Work out the finished part from the listing and answer in its coordinate system (mm). Face numbers are marked on the shaded views. Give positions to 0.01 mm unless a question says otherwise; leave off trailing zeros. Loops run counter-clockwise (first coordinate to the right, second up) from the corner with the lowest first, then second, coordinate; pieces in that order, holes last.
```python
from build123d import *

# Parameters (mm, degrees)
BOX028_W          = 10
BOX028_H          = 10
BOX028_DEPTH      = 3.5
FILLET018_R       = 1.7
BOX029_W          = 20
BOX029_H          = 10
BOX029_DEPTH      = 3.5
FILLET019_R       = 1.7
CYLINDER029_R     = 5
CYLINDER029_DEPTH = 10
CYLINDER027_R     = 0.25
CYLINDER027_DEPTH = 10
CYLINDER026_R     = 1.75
CYLINDER026_DEPTH = 10
BOX023_W          = 6.65
BOX023_H          = 8.3
BOX023_DEPTH      = 2.45
FILLET014_R       = 1
CYLINDER022_R     = 0.5
CYLINDER022_DEPTH = 10
CYLINDER023_R     = 0.5
CYLINDER023_DEPTH = 10
CYLINDER024_R     = 0.5
CYLINDER024_DEPTH = 10
CYLINDER021_R     = 0.5
CYLINDER021_DEPTH = 10
CYLINDER020_R     = 0.5
CYLINDER020_DEPTH = 10
CYLINDER019_R     = 0.5
CYLINDER019_DEPTH = 10
CYLINDER018_R     = 0.5
CYLINDER018_DEPTH = 10
CYLINDER017_R     = 0.5
CYLINDER017_DEPTH = 10
CYLINDER016_R     = 0.5
CYLINDER016_DEPTH = 10
CYLINDER015_R     = 0.5
CYLINDER015_DEPTH = 10
CYLINDER014_R     = 0.5
CYLINDER014_DEPTH = 10
CYLINDER013_R     = 0.5
CYLINDER013_DEPTH = 10
BOX021_W          = 8
BOX021_H          = 4
BOX021_DEPTH      = 10
FILLET012_R       = 1.5
BOX019_W          = 8
BOX019_H          = 8
BOX019_DEPTH      = 10
FILLET010_R       = 3
BOX001_W          = 133
BOX001_H          = 63
BOX001_DEPTH      = 10
FILLET002_R       = 1
BOX_W             = 137
BOX_H             = 67
BOX_DEPTH         = 7.5
FILLET_R          = 3
FILLET001_R       = 2


with BuildPart() as fillet018:
    # Box028 → Box028 (new body)
    with BuildSketch(Plane(origin=(57, 60, 2.5), x_dir=(1, 0, 0), z_dir=(0, 0, 1))):
        with Locations((5, 5)):
            Rectangle(BOX028_W, BOX028_H)
    extrude(amount=BOX028_DEPTH)

    # Fillet018
    fillet018_edges = [fillet018.edges().sort_by_distance(p)[0] for p in [
        (57, 65, 6),
        (57, 65, 2.5),
        (67, 65, 6),
        (67, 65, 2.5),
    ]]
    fillet(fillet018_edges, radius=FILLET018_R)


with BuildPart() as fillet018_1:
    # Fillet018 placement: moved
    add(fillet018.part.moved(Location((0, 0, -0.6))))


with BuildPart() as fillet019:
    # Box029 → Box029 (new body)
    with BuildSketch(Plane(origin=(57, 60, 2.5), x_dir=(1, 0, 0), z_dir=(0, 0, 1))):
        with Locations((10, 5)):
            Rectangle(BOX029_W, BOX029_H)
    extrude(amount=BOX029_DEPTH)

    # Fillet019
    fillet019_edges = [fillet019.edges().sort_by_distance(p)[0] for p in [
        (57, 65, 6),
        (57, 65, 2.5),
        (77, 65, 6),
        (77, 65, 2.5),
    ]]
    fillet(fillet019_edges, radius=FILLET019_R)


with BuildPart() as fillet019_1:
    # Fillet019 placement: moved
    add(fillet019.part.moved(Location((-25, 0, -0.6))))


with BuildPart() as cilindro027:
    # Cylinder029 → Cylinder029 (new body)
    with BuildSketch(Plane(origin=(37, 33.5, -1), x_dir=(1, 0, 0), z_dir=(0, 0, 1))):
        Circle(CYLINDER029_R)
    extrude(amount=CYLINDER029_DEPTH)


with BuildPart() as cilindro025:
    # Cylinder027 → Cylinder027 (new body)
    with BuildSketch(Plane(origin=(0, 16, 3), x_dir=(0, 1, 0), z_dir=(1, 0, 0))):
        Circle(CYLINDER027_R)
    extrude(amount=CYLINDER027_DEPTH)


with BuildPart() as phones:
    # Cylinder026 → Cylinder026 (new body)
    with BuildSketch(Plane(origin=(-2, 11.75, 3), x_dir=(0, 1, 0), z_dir=(1, 0, 0))):
        Circle(CYLINDER026_R)
    extrude(amount=CYLINDER026_DEPTH)


with BuildPart() as usb_c:
    # Box023 → Box023 (new body)
    with BuildSketch(Plane.XY):
        with Locations((3.325, 4.15)):
            Rectangle(BOX023_W, BOX023_H)
    extrude(amount=BOX023_DEPTH)

    # Fillet014
    fillet014_edges = [usb_c.edges().sort_by_distance(p)[0] for p in [
        (3.325, 0, 0),
        (3.325, 0, 2.45),
        (3.325, 8.3, 0),
        (3.325, 8.3, 2.45),
    ]]
    fillet(fillet014_edges, radius=FILLET014_R)


with BuildPart() as usb_c_1:
    # Fillet014 placement: moved
    add(usb_c.part.moved(Location((132, 29.35, 2.4))))


with BuildPart() as cilindro022:
    # Cylinder022 → Cylinder022 (new body)
    with BuildSketch(Plane(origin=(130, 52.5, 4.25), x_dir=(0, 1, 0), z_dir=(1, 0, 0))):
        Circle(CYLINDER022_R)
    extrude(amount=CYLINDER022_DEPTH)


with BuildPart() as cilindro023:
    # Cylinder023 → Cylinder023 (new body)
    with BuildSketch(Plane(origin=(130, 51, 4.25), x_dir=(0, 1, 0), z_dir=(1, 0, 0))):
        Circle(CYLINDER023_R)
    extrude(amount=CYLINDER023_DEPTH)


with BuildPart() as fusion008:
    # Cylinder024 → Cylinder024 (new body)
    with BuildSketch(Plane(origin=(130, 54, 4.25), x_dir=(0, 1, 0), z_dir=(1, 0, 0))):
        Circle(CYLINDER024_R)
    extrude(amount=CYLINDER024_DEPTH)

    # Fusion009: union Cilindro022, Cilindro023
    add(cilindro022.part)
    add(cilindro023.part)


with BuildPart() as fusion008_1:
    # Fusion009 placement: moved
    add(fusion008.part.moved(Location((0, -33.5, 0))))


with BuildPart() as cilindro021:
    # Cylinder021 → Cylinder021 (new body)
    with BuildSketch(Plane(origin=(130, 52.5, 4.25), x_dir=(0, 1, 0), z_dir=(1, 0, 0))):
        Circle(CYLINDER021_R)
    extrude(amount=CYLINDER021_DEPTH)


with BuildPart() as cilindro020:
    # Cylinder020 → Cylinder020 (new body)
    with BuildSketch(Plane(origin=(130, 51, 4.25), x_dir=(0, 1, 0), z_dir=(1, 0, 0))):
        Circle(CYLINDER020_R)
    extrude(amount=CYLINDER020_DEPTH)


with BuildPart() as agujero_micro:
    # Cylinder019 → Cylinder019 (new body)
    with BuildSketch(Plane(origin=(130, 54, 4.25), x_dir=(0, 1, 0), z_dir=(1, 0, 0))):
        Circle(CYLINDER019_R)
    extrude(amount=CYLINDER019_DEPTH)

    # Fusion008: union Cilindro021, Cilindro020
    add(cilindro021.part)
    add(cilindro020.part)


with BuildPart() as agujero_micro_1:
    # Fusion008 placement: moved
    add(agujero_micro.part.moved(Location((0, -38, 0))))

    # Fusion010: union Fusion008
    add(fusion008_1.part)


with BuildPart() as cilindro018:
    # Cylinder018 → Cylinder018 (new body)
    with BuildSketch(Plane(origin=(130, 52.5, 4.25), x_dir=(0, 1, 0), z_dir=(1, 0, 0))):
        Circle(CYLINDER018_R)
    extrude(amount=CYLINDER018_DEPTH)


with BuildPart() as cilindro017:
    # Cylinder017 → Cylinder017 (new body)
    with BuildSketch(Plane(origin=(130, 51, 4.25), x_dir=(0, 1, 0), z_dir=(1, 0, 0))):
        Circle(CYLINDER017_R)
    extrude(amount=CYLINDER017_DEPTH)


with BuildPart() as fusion006:
    # Cylinder016 → Cylinder016 (new body)
    with BuildSketch(Plane(origin=(130, 54, 4.25), x_dir=(0, 1, 0), z_dir=(1, 0, 0))):
        Circle(CYLINDER016_R)
    extrude(amount=CYLINDER016_DEPTH)

    # Fusion006: union Cilindro018, Cilindro017
    add(cilindro018.part)
    add(cilindro017.part)


with BuildPart() as fusion006_1:
    # Fusion006 placement: moved
    add(fusion006.part.moved(Location((0, -4.5, 0))))


with BuildPart() as cilindro015:
    # Cylinder015 → Cylinder015 (new body)
    with BuildSketch(Plane(origin=(130, 52.5, 4.25), x_dir=(0, 1, 0), z_dir=(1, 0, 0))):
        Circle(CYLINDER015_R)
    extrude(amount=CYLINDER015_DEPTH)


with BuildPart() as cilindro014:
    # Cylinder014 → Cylinder014 (new body)
    with BuildSketch(Plane(origin=(130, 51, 4.25), x_dir=(0, 1, 0), z_dir=(1, 0, 0))):
        Circle(CYLINDER014_R)
    extrude(amount=CYLINDER014_DEPTH)


with BuildPart() as obj1:
    # Cylinder013 → Cylinder013 (new body)
    with BuildSketch(Plane(origin=(130, 54, 4.25), x_dir=(0, 1, 0), z_dir=(1, 0, 0))):
        Circle(CYLINDER013_R)
    extrude(amount=CYLINDER013_DEPTH)

    # Fusion005: union Cilindro015, Cilindro014
    add(cilindro015.part)
    add(cilindro014.part)

    # Fusion007: union Fusion006
    add(fusion006_1.part)


with BuildPart() as fillet012:
    # Box021 → Box021 (new body)
    with BuildSketch(Plane(origin=(4, 55, -1), x_dir=(1, 0, 0), z_dir=(0, 0, 1))):
        with Locations((4, 2)):
            Rectangle(BOX021_W, BOX021_H)
    extrude(amount=BOX021_DEPTH)

    # Fillet012
    fillet012_edges = [fillet012.edges().sort_by_distance(p)[0] for p in [
        (4, 55, 4),
        (4, 59, 4),
        (12, 55, 4),
        (12, 59, 4),
    ]]
    fillet(fillet012_edges, radius=FILLET012_R)


with BuildPart() as fillet012_1:
    # Fillet012 placement: moved
    add(fillet012.part.moved(Location((0, -6, 0))))


with BuildPart() as fillet010:
    # Box019 → Box019 (new body)
    with BuildSketch(Plane(origin=(4, 55, -1), x_dir=(1, 0, 0), z_dir=(0, 0, 1))):
        with Locations((4, 4)):
            Rectangle(BOX019_W, BOX019_H)
    extrude(amount=BOX019_DEPTH)

    # Fillet010
    fillet010_edges = [fillet010.edges().sort_by_distance(p)[0] for p in [
        (4, 55, 4),
        (4, 63, 4),
        (12, 55, 4),
        (12, 63, 4),
    ]]
    fillet(fillet010_edges, radius=FILLET010_R)


with BuildPart() as fillet002:
    # Box001 → Box001 (new body)
    with BuildSketch(Plane(origin=(2, 2, 5.5), x_dir=(1, 0, 0), z_dir=(0, 0, 1))):
        with Locations((66.5, 31.5)):
            Rectangle(BOX001_W, BOX001_H)
    extrude(amount=BOX001_DEPTH)

    # Fillet002
    fillet002_edges = [fillet002.edges().sort_by_distance(p)[0] for p in [
        (2, 2, 10.5),
        (2, 65, 10.5),
        (135, 2, 10.5),
        (135, 65, 10.5),
    ]]
    fillet(fillet002_edges, radius=FILLET002_R)


with BuildPart() as fillet002_1:
    # Fillet002 placement: moved
    add(fillet002.part.moved(Location((0, 0, -4.5))))


with BuildPart() as cut037:
    # Box → Box (new body)
    with BuildSketch(Plane.XY):
        with Locations((68.5, 33.5)):
            Rectangle(BOX_W, BOX_H)
    extrude(amount=BOX_DEPTH)

    # Fillet
    fillet_edges = [cut037.edges().sort_by_distance(p)[0] for p in [
        (0, 0, 3.75),
        (0, 67, 3.75),
        (0, 33.5, 0),
        (137, 0, 3.75),
        (137, 67, 3.75),
        (137, 33.5, 0),
        (68.5, 0, 0),
        (68.5, 67, 0),
    ]]
    fillet(fillet_edges, radius=FILLET_R)

    # Fillet001
    fillet001_edges = [cut037.edges().sort_by_distance(p)[0] for p in [
        (0, 33.5, 7.5),
        (0.87868, 0.87868, 7.5),
        (68.5, 0, 7.5),
        (68.5, 67, 7.5),
        (136.12132, 0.87868, 7.5),
        (136.12132, 66.12132, 7.5),
        (137, 33.5, 7.5),
    ]]
    fillet(fillet001_edges, radius=FILLET001_R)

    # Cut: cut Fillet002
    add(fillet002_1.part, mode=Mode.SUBTRACT)

    # Cut024: cut Fillet010
    add(fillet010.part, mode=Mode.SUBTRACT)

    # Cut025: cut Fillet012
    add(fillet012_1.part, mode=Mode.SUBTRACT)

    # Cut026: cut obj1
    add(obj1.part, mode=Mode.SUBTRACT)

    # Cut027: cut Agujero Micro
    add(agujero_micro_1.part, mode=Mode.SUBTRACT)

    # Cut028: cut USB-C
    add(usb_c_1.part, mode=Mode.SUBTRACT)

    # Cut029: cut phones
    add(phones.part, mode=Mode.SUBTRACT)

    # Cut031: cut Cilindro025
    add(cilindro025.part, mode=Mode.SUBTRACT)

    # Cut034: cut Cilindro027
    add(cilindro027.part, mode=Mode.SUBTRACT)

    # Cut036: cut Fillet019
    add(fillet019_1.part, mode=Mode.SUBTRACT)

    # Cut037: cut Fillet018
    add(fillet018_1.part, mode=Mode.SUBTRACT)


solid = cut037.part
```
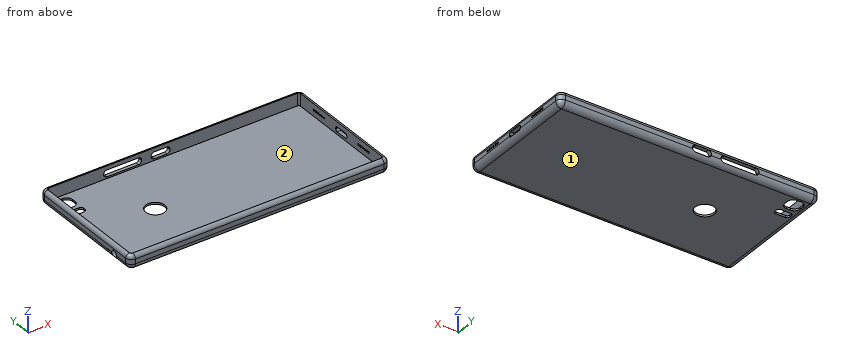
Q1. Section C-C on x = 123.5 is taken. Give the vertices of the cut face in (y, z), plus the area to 3 significant figures.
Q2. Section A-A on x = 37 is taken. Give the vertices of the cut face in (y, z), plus the area to 3 significant figures.
Q3. Determine the mould class of the marked faces 1 and 2 for opening direction X: +X half, -X half, draft (parallel to the pull), parting line (faces both ways), or undercut.
Q4. Consider line 1 along Y through (x, z) = (20, 5.5); line 2 along X through (y, z) = (44, 3.5); line 3 along Z through (x, y) = (25.5, 23.5). Determine where each line is inside the solid, lowest interval first.
Q5. Section B-B on y = 7.5 is taken. Give the vertices of the cut face in (x, z), plus the area to 3 significant figures.
Q6. Given pin 1 (0.5 mm diameter, centred on x = 62.5, y = 66, fed in from +Z); pin 2 (2 mm diameter, centred on x = 14.5, y = 60, fed in from +Z); pin 3 (0.5 mm diameter, centred on x = 8.5, z = 0.5, fed in from -Y), each flat-ended and moving along its own axis, determine where each tip first touches the part or whether it passes through.
Check result:
1. outline: (0, 3) arc R3 ccw to (3, 0) - (64, 0) arc R3 ccw to (67, 3) - (67, 5.5) arc R2 ccw to (65, 7.5) - (65, 1) - (2, 1) - (2, 7.5) arc R2 ccw to (0, 5.5) - close
1. area: 87.4 mm2
2. outline: (0, 3) arc R3 ccw to (3, 0) - (28.5, 0) - (28.5, 1) - (2, 1) - (2, 7.5) arc R2 ccw to (0, 5.5) - close; (38.5, 0) - (64, 0) arc R3 ccw to (66.79, 1.9) - (65, 1.9) - (65, 1) - (38.5, 1) - close; (65, 5.4) - (67, 5.4) - (67, 5.5) arc R2 ccw to (65, 7.5) - close
2. area: 70.5 mm2
3. face 1: draft
3. face 2: undercut
4. line 1: y = 0 to 2, 65 to 67
4. line 2: x = 0 to 2, 135 to 137
4. line 3: z = 0 to 1
5. outline: (0, 3) arc R3 ccw to (3, 0) - (134, 0) arc R3 ccw to (137, 3) - (137, 5.5) arc R2 ccw to (135, 7.5) - (135, 1) - (2, 1) - (2, 7.5) arc R2 ccw to (0, 5.5) - close
5. area: 157 mm2
6. pin 1: stops at z = 7.35
6. pin 2: stops at z = 1
6. pin 3: stops at y = 1.02
